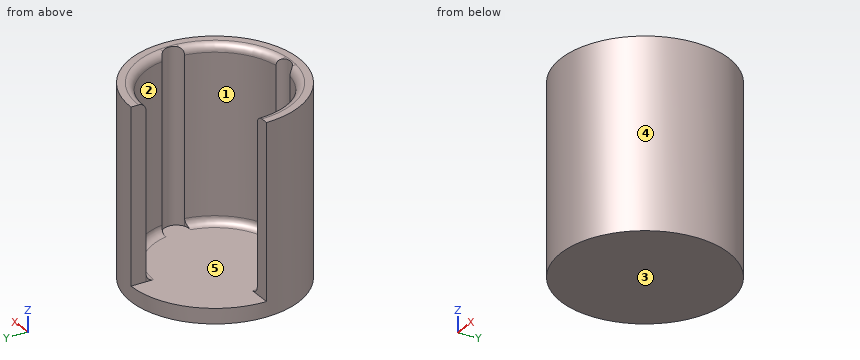
from build123d import *

# Parameters (mm, degrees)
F0_R         = 11.15
F1_DEPTH     = 25
F3_DEPTH     = 23
F4_T4_ANGLE  = 102.4463467312
F4_S5_R      = 1.65
F4_T6_DEPTH  = 9
F4_S7_R      = 1.65
F4_T8_DEPTH  = 9
F4_T12_ANGLE = 96.2242847007
F4_S13_R     = 1.65
F4_T14_DEPTH = 9
F4_T18_ANGLE = 96.2242847007
F4_S19_R     = 1.65
F4_T20_DEPTH = 9
F4_T22_ANGLE = 102.4463467312
F4_T24_ANGLE = 111.8839081247
F4_T26_ANGLE = 111.8839081247


# Not quite as in the source:
# - a fillet or chamfer that OpenCascade refuses, or shapes differently, is made with other operations: its cross-section is extruded or revolved along the edge and cut away or added


with BuildPart() as f1:
    # F0 (on Top) → F1 (new body)
    with BuildSketch(Plane.XY):
        Circle(F0_R)
    extrude(amount=F1_DEPTH)

    # F2 (on face) → F3 (cut)
    with BuildSketch(Plane.XY.offset(25)):
        with BuildLine():
            ThreePointArc((9.02621183, -1.5), (9.1190004453, -0.7525495849), (9.15, 0))
            ThreePointArc((9.15, 0), (9.1190004453, 0.7525495849), (9.02621183, 1.5))
            ThreePointArc((9.02621183, 1.5), (5.9159741379, 6.9802399672), (0, 9.15))
            ThreePointArc((0, 9.15), (-6.4700270479, 6.4700270479), (-9.15, 0))
            ThreePointArc((-9.15, 0), (-6.9802399672, -5.9159741379), (-1.5, -9.02621183))
            ThreePointArc((-1.5, -9.02621183), (0, -9.15), (1.5, -9.02621183))
            ThreePointArc((1.5, -9.02621183), (6.4700270479, -6.4700270479), (9.02621183, -1.5))
        make_face()
        with BuildLine():
            ThreePointArc((9.02621183, 1.5), (9.1190004453, 0.7525495849), (9.15, 0))
            ThreePointArc((9.15, 0), (9.1190004453, -0.7525495849), (9.02621183, -1.5))
            ThreePointArc((9.02621183, -1.5), (9.9888254758, 0), (9.02621183, 1.5))
        make_face()
        with BuildLine():
            ThreePointArc((-1.5, -9.02621183), (0, -9.9888254758), (1.5, -9.02621183))
            ThreePointArc((1.5, -9.02621183), (0, -9.15), (-1.5, -9.02621183))
        make_face()
        with BuildLine():
            ThreePointArc((-9.15, 0), (-6.4700270479, 6.4700270479), (0, 9.15))
            Line((0, 9.15), (0, 11.15))
            ThreePointArc((0, 11.15), (-7.8842406102, 7.8842406102), (-11.15, 0))
            Line((-11.15, 0), (-9.15, 0))
        make_face()
    extrude(amount=-F3_DEPTH, mode=Mode.SUBTRACT)

    # F4: fillet of radius 1 on 6 edges, made by hand


with BuildPart() as f4_tool2:
    # F4_s3 → F4_t4 (revolve)
    with BuildSketch(Plane(origin=(0, 0, 0), x_dir=(0, 0, 1), z_dir=(-0.9941072022, 0.1084014327, 0))):
        with BuildLine():
            ThreePointArc((2, -8.15), (2.2928932188, -8.8571067812), (3, -9.15))
            Line((3, -9.15), (2, -9.15))
            Line((2, -9.15), (2, -8.15))
        make_face()
    revolve(axis=Axis((0, 0, 2), (0, 0, 1)), revolution_arc=F4_T4_ANGLE)

    # F4_s5 → F4_t6 (cut, symmetric)
    with BuildSketch(Plane.XY.offset(2.9)):
        with Locations((8.3388254758, 0)):
            Circle(F4_S5_R)
    extrude(amount=F4_T6_DEPTH, both=True, mode=Mode.SUBTRACT)

    # F4_s7 → F4_t8 (cut, symmetric)
    with BuildSketch(Plane.XY.offset(2.9)):
        with Locations((0, -8.3388254758)):
            Circle(F4_S7_R)
    extrude(amount=F4_T8_DEPTH, both=True, mode=Mode.SUBTRACT)


with BuildPart() as f1_1:
    add(f1.part)

    # F4_t1: union F4_tool2
    add(f4_tool2.part)


with BuildPart() as f4_tool10:
    # F4_s11 → F4_t12 (revolve)
    with BuildSketch(Plane(origin=(0, 0, 0), x_dir=(0, 0, 1), z_dir=(-0.1084207149, -0.9941050994, 0))):
        with BuildLine():
            ThreePointArc((2, -8.15), (2.2928932188, -8.8571067812), (3, -9.15))
            Line((3, -9.15), (2, -9.15))
            Line((2, -9.15), (2, -8.15))
        make_face()
    revolve(axis=Axis((0, 0, 2), (0, 0, 1)), revolution_arc=F4_T12_ANGLE)

    # F4_s13 → F4_t14 (cut, symmetric)
    with BuildSketch(Plane.XY.offset(2.9)):
        with Locations((8.3388254758, 0)):
            Circle(F4_S13_R)
    extrude(amount=F4_T14_DEPTH, both=True, mode=Mode.SUBTRACT)


with BuildPart() as f1_2:
    add(f1_1.part)

    # F4_t9: union F4_tool10
    add(f4_tool10.part)


with BuildPart() as f4_tool16:
    # F4_s17 → F4_t18 (revolve)
    with BuildSketch(Plane.XZ):
        with BuildLine():
            ThreePointArc((-8.15, 2), (-8.8571067812, 2.2928932188), (-9.15, 3))
            Line((-9.15, 3), (-9.15, 2))
            Line((-9.15, 2), (-8.15, 2))
        make_face()
    revolve(axis=Axis((0, 0, 2), (0, 0, 1)), revolution_arc=F4_T18_ANGLE)

    # F4_s19 → F4_t20 (cut, symmetric)
    with BuildSketch(Plane.XY.offset(2.9)):
        with Locations((0, -8.3388254758)):
            Circle(F4_S19_R)
    extrude(amount=F4_T20_DEPTH, both=True, mode=Mode.SUBTRACT)


with BuildPart() as f1_3:
    add(f1_2.part)

    # F4_t15: union F4_tool16
    add(f4_tool16.part)

    # F4_s21 → F4_t22 (revolve, cut)
    with BuildSketch(Plane(origin=(0, 0, 0), x_dir=(0, 0, 1), z_dir=(-0.9941072022, 0.1084014327, 0))):
        with BuildLine():
            ThreePointArc((24, -9.15), (24.7071067812, -9.4428932188), (25, -10.15))
            Line((25, -10.15), (25, -9.15))
            Line((25, -9.15), (24, -9.15))
        make_face()
    revolve(axis=Axis((0, 0, 25), (0, 0, 1)), revolution_arc=F4_T22_ANGLE, mode=Mode.SUBTRACT)

    # F4_s23 → F4_t24 (revolve, cut)
    with BuildSketch(Plane(origin=(0, 0, 0), x_dir=(0, 0, 1), z_dir=(0.2699219659, 0.9628822006, 0))):
        with BuildLine():
            ThreePointArc((24, -9.15), (24.7071067812, -9.4428932188), (25, -10.15))
            Line((25, -10.15), (25, -9.15))
            Line((25, -9.15), (24, -9.15))
        make_face()
    revolve(axis=Axis((0, 0, 25), (0, 0, 1)), revolution_arc=F4_T24_ANGLE, mode=Mode.SUBTRACT)

    # F4_s25 → F4_t26 (revolve, cut)
    with BuildSketch(Plane(origin=(0, 0, 0), x_dir=(0, 0, 1), z_dir=(-0.1084207149, -0.9941050994, 0))):
        with BuildLine():
            ThreePointArc((24, -9.15), (24.7071067812, -9.4428932188), (25, -10.15))
            Line((25, -10.15), (25, -9.15))
            Line((25, -9.15), (24, -9.15))
        make_face()
    revolve(axis=Axis((0, 0, 25), (0, 0, 1)), revolution_arc=F4_T26_ANGLE, mode=Mode.SUBTRACT)


solid = f1_3.part
CAD build for the part. Positions are in the model's coordinates, mm. Face numbers are marked on the shaded views. A direction names the side the tool comes from. Give positions to 0.01 mm unless a question says otherwise; leave off trailing zeros. Write each loop counter-clockwise with the first axis right and the second up, starting at its lowest first coordinate (ties: lowest second). Pieces come first, ordered by that corner, then holes. Notation, with made-up numbers: (61.25, -12.75) -> (70.25, -12.75) arc R13 cw to (70.25, 9.25) -> close; hole circle Ø10 at (19, 89). An arc over 180 degrees is marked (long way). Return JSON: item names as keys, results as strings.
Item 1: Drill centre lines: probe 1 along Z at (x, y) = (4.5, 0.75); probe 2 along Z at (x, y) = (-1.25, -10); probe 3 along X at (y, z) = (-4.5, 14.75). Where is each one in solid material? Low to high.
Answer below:
{"probe 1": "z = 0 to 2", "probe 2": "z = 0 to 25", "probe 3": "x = -10.2 to -7.97, 7.97 to 10.2"}
Item 2: Two-plate mould, pull along X, no slides. Class the marked faces 3, 4 and 5: +X half, -X half, draft (parallel to the pull), parting line (faces both ways), or undercut.
Answer below:
{"face 3": "draft", "face 4": "parting line", "face 5": "undercut"}
Item 3: Drop flat-ended pins along their axis: pin 1 (1 mm diameter, centred on y = 5, z = 22.5, fed in from -X); pin 2 (3.5 mm diameter, centred on x = -10, z = 16.5, fed in from +Y); pin 3 (6 mm diameter, centred on y = -8.5, z = 18, fed in from -X). Give the stop position or say it passes through.
Answer below:
{"pin 1": "stops at x = 7.31", "pin 2": "stops at y = 0", "pin 3": "stops at x = -9.7"}
Item 4: Tool access for the marked faces 1 and 2: list every direction of +Z, -Z, +X, -X, +Y, -Y with a clear straight run to the whole face (end or side of a thin tool).
Answer below:
{"face 1": "+Z", "face 2": "+Z, -X"}
Item 5: Band-saw the part on A-A (z = 21.5). List the corners of the cut face in (x, y).
Answer below:
{"outline": "(-11.15, 0) arc R11.15 ccw (long way) to (0, 11.15) -> (0, 9.15) arc R9.15 cw to (9.03, 1.5) arc R1.65 cw to (9.03, -1.5) arc R9.15 cw to (1.5, -9.03) arc R1.65 cw to (-1.5, -9.03) arc R9.15 cw to (-9.15, 0) -> close"}
